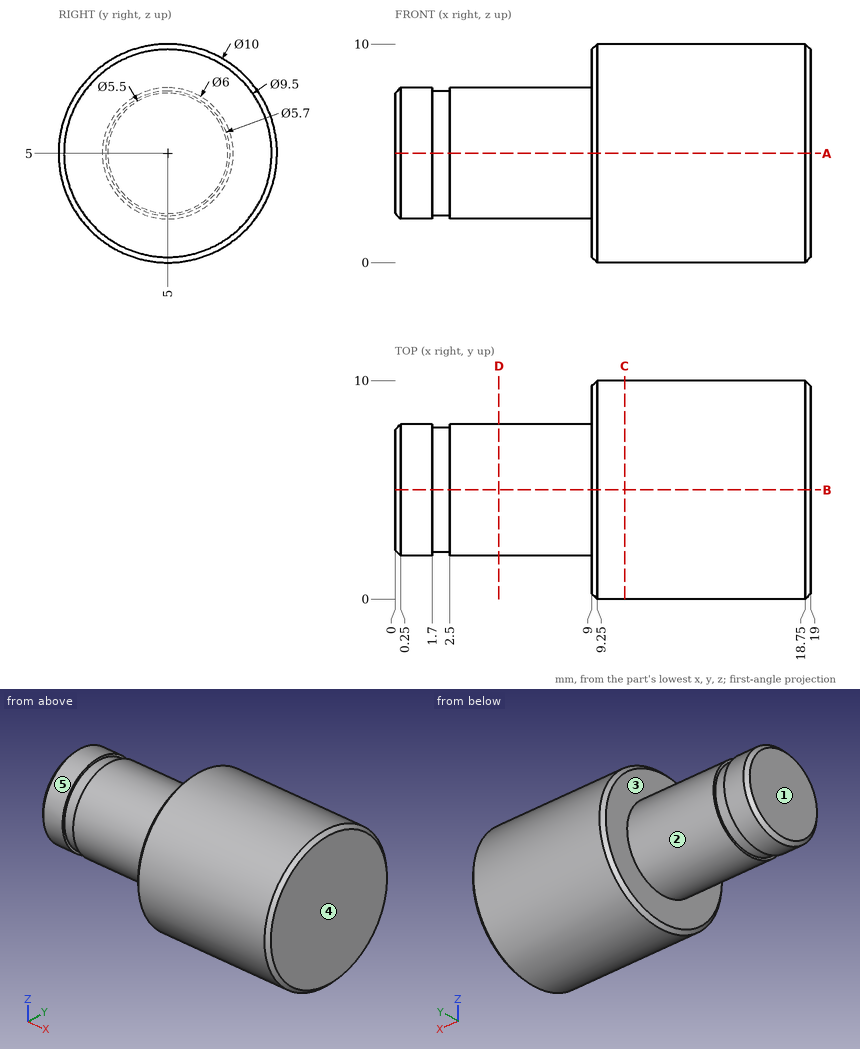
Input: dimensioned drawing with shaded views. Units: mm. Origin: part minimum x, y, z. A direction names the side the tool comes from. Round coordinates to 2 decimals unless told otherwise and drop trailing zeros. Order: outer loops, then holes, each group sorted by start corner. A loop starts at its lowest first (then second) coordinate and runs counter-clockwise, first axis right, second up. Notation, with made-up numbers: (12.5, 79) - (64.5, 79) arc R15 ccw to (64.5, 87) - close; hole circle Ø3 at (-14.5, 24). An arc over 180 degrees is marked (long way). Write item = value, one per line. Start each with the question number.
Q1. Access query for the marked faces 1 and 2. Directions: +Z, -Z, +X, -X, +Y, -Y. A direction counts if a zero-diameter tool reaches every point of the face in a straight line with its end or side. Return the directions, or none.
Q2. Cut plane C-C on x = 10.5. Return the cut outline in (y, z).
Q3. Cut plane D-D on x = 4.75. Return the cut outline in (y, z), and give its area (3 significant figures).
Q4. Pin query (flat end, axial travel): pin 1 (1.8 mm diameter, centred on y = 5.5, z = 4, fed in from -X); pin 2 (1.5 mm diameter, centred on x = 5, y = 4.5, fed in from +Z); pin 3 (3 mm diameter, centred on x = 12.5, y = 7, fed in from -Z); pin 4 (3 mm diameter, centred on x = 14.5, z = 7.5, fed in from +Y). Return the tip coordinate at first contact, or that it passes through.
Q5. Ray query, line 1 (X direction, y = 9.5, z = 4.5); line 2 (Z direction, x = 4, y = 5); line 3 (Y direction, x = 11.75, z = 2.5). Return the intervals inside material, ascending. Write a range as from..to.
Q6. Cut plane A-A on z = 5. Return the cut outline in (x, y), and give its area (3 significant figures).
Q7. Pull-direction query (X, two-part tool) for the marked faces 3, 4 and 5; classes: +X half, -X half, draft (parallel to the pull), parting line (faces both ways), or undercut.
Outcome:
q1.face_1 = +Z, -Z, -X, +Y, -Y
q1.face_2 = -X
q2.outline = circle Ø10 at (5, 5)
q3.outline = circle Ø6 at (5, 5)
q3.area = 28.3 mm^2
q4.pin_1 = 0
q4.pin_2 = 8
q4.pin_3 = 0.03
q4.pin_4 = 9.9
q5.line_1 = 9..19
q5.line_2 = 2..8
q5.line_3 = 0.67..9.33
q6.outline = (0, 2.25) - (0.25, 2) - (1.7, 2) - (1.7, 2.15) - (2.5, 2.15) - (2.5, 2) - (9, 2) - (9, 0.25) - (9.25, 0) - (18.75, 0) - (19, 0.25) - (19, 9.75) - (18.75, 10) - (9.25, 10) - (9, 9.75) - (9, 8) - (2.5, 8) - (2.5, 7.85) - (1.7, 7.85) - (1.7, 8) - (0.25, 8) - (0, 7.75) - close
q6.area = 154 mm^2
q7.face_3 = -X half
q7.face_4 = +X half
q7.face_5 = draft
